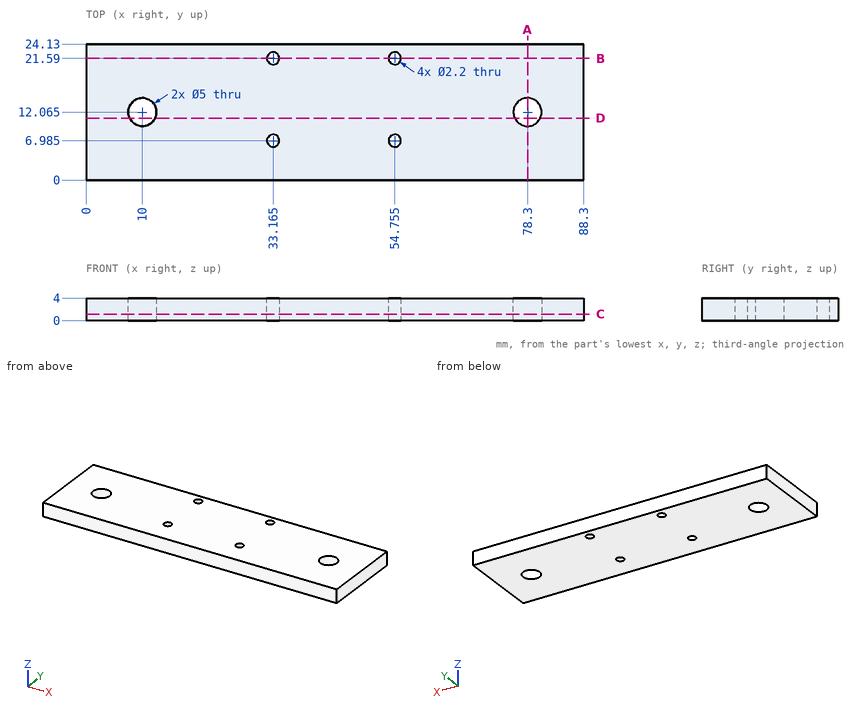
The drawing under review shows one solid part. Ordinate dimensions are in mm from its lowest x, y, z. Coordinates: 2 decimals unless noted, no trailing zeros. Write each loop counter-clockwise with the first axis right and the second up, starting at its lowest first coordinate (ties: lowest second). Pieces come first, ordered by that corner, then holes.
1) Add section C-C (z = 1.15). Write out the cut boundary in (x, y) (1 decimal).
2) Insertion check: pin 1 (10 mm diameter, centred on x = 58.5, y = 21.5, fed in from -Z). The pin has a flat end and moves straight along its axis. Give the tip position at first contact, or say it passes through.
3) Add section B-B (y = 21.59). Write out the cut boundary in (x, z) (1 decimal).
4) Add section A-A (x = 78.3). Write out the cut boundary in (y, z) (1 decimal).
5) To check wall thickness, follow L1, parallel to X at y = 12, z = 2; L2, parallel to X at y = 21, z = 2.7 (1 decimal); L3, parallel to Y at x = 77, z = 2.05. State the ranges of each line that lie inside material, in increasing order.
6) Add section D-D (y = 11). Write out the cut boundary in (x, z).
Check result:
1. outline: (0, 0) - (88.3, 0) - (88.3, 24.1) - (0, 24.1) - close; hole circle Ø5 at (10, 12.1); hole circle Ø2.2 at (33.2, 7); hole circle Ø2.2 at (33.2, 21.6); hole circle Ø2.2 at (54.8, 7); hole circle Ø2.2 at (54.8, 21.6); hole circle Ø5 at (78.3, 12.1)
2. pin 1: stops at z = 0
3. outline: (0, 0) - (32.1, 0) - (32.1, 4) - (0, 4) - close; (34.3, 0) - (53.7, 0) - (53.7, 4) - (34.3, 4) - close; (55.9, 0) - (88.3, 0) - (88.3, 4) - (55.9, 4) - close
4. outline: (0, 0) - (9.6, 0) - (9.6, 4) - (0, 4) - close; (14.6, 0) - (24.1, 0) - (24.1, 4) - (14.6, 4) - close
5. L1: x = 0 to 7.5, 12.5 to 75.8, 80.8 to 88.3
5. L2: x = 0 to 32.2, 34.1 to 53.8, 55.7 to 88.3
5. L3: y = 0 to 9.93, 14.2 to 24.13
6. outline: (0, 0) - (7.74, 0) - (7.74, 4) - (0, 4) - close; (12.26, 0) - (76.04, 0) - (76.04, 4) - (12.26, 4) - close; (80.56, 0) - (88.3, 0) - (88.3, 4) - (80.56, 4) - close
